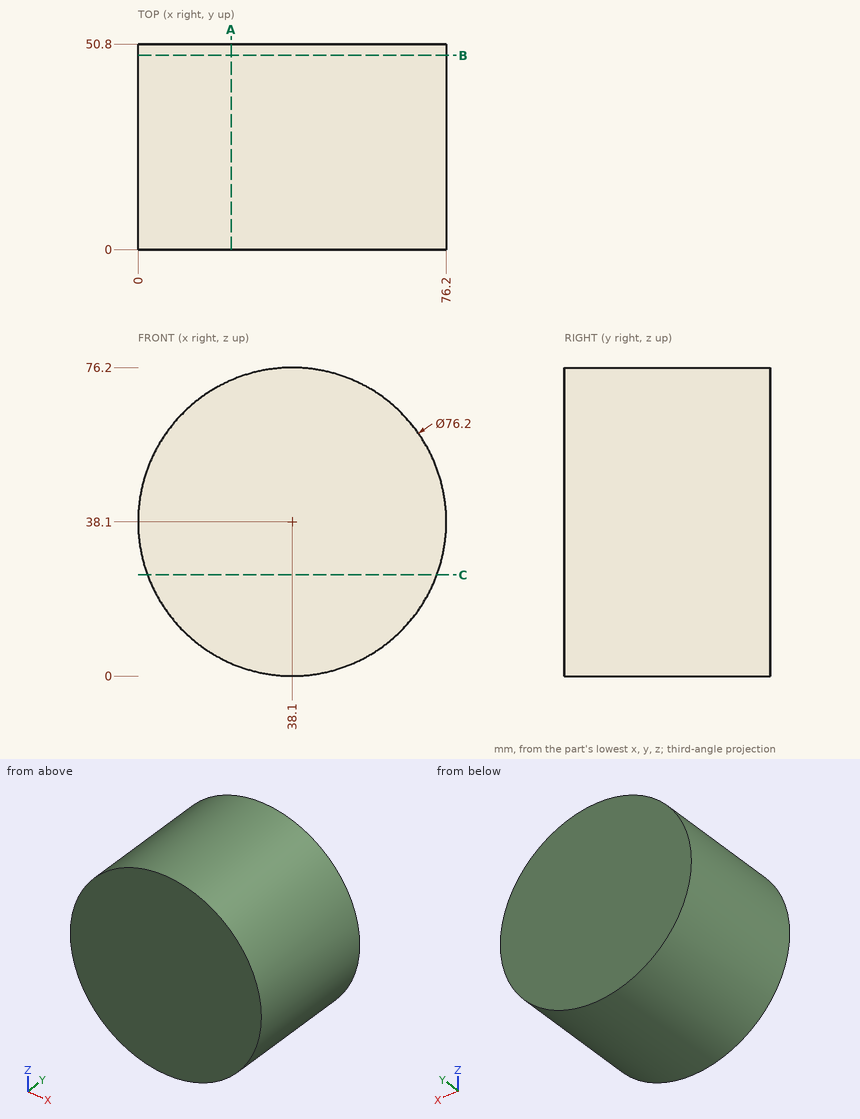
Verification items for this drawing (mm, ordinates from the low corner). Coordinates: 2 decimals unless noted, no trailing zeros. Order: outer loops, then holes, each group sorted by start corner. A loop starts at its lowest first (then second) coordinate and runs counter-clockwise, first axis right, second up. Notation, with made-up numbers: M -0.75,6.5 L 45.25,6.5 A14 ccw 45.25,26.5 Z; hole C 80.5,4.5 d10. An arc over 180 degrees is marked long. Use CSV: the item, a comma, the result in double quotes.
Item 1: Cross-section at A-A on x = 23. Record the cut outline in (y, z), then the cut area to 3 significant figures.
Returned:
outline,"M 0,3.12 L 50.8,3.12 L 50.8,73.08 L 0,73.08 Z"
area,"3,550 mm2"
Item 2: Gauge pin test, flat ends, axial feed: pin 1 Ø1.5 at (y, z) = (16, 63.5) entering from +X; pin 2 Ø2 at (y, z) = (5.5, 30.5) entering from +X; pin 3 Ø8 at (x, y) = (38, 5) entering from -Z. Record the tip position at first contact, or that the pin passes through.
Returned:
pin 1,"stops at x = 67.15"
pin 2,"stops at x = 75.62"
pin 3,"stops at z = 0"
Item 3: Cross-section at C-C on z = 25. Record the cut outline in (x, y).
Returned:
outline,"M 2.32,0 L 73.88,0 L 73.88,50.8 L 2.32,50.8 Z"
Item 4: Cross-section at B-B on y = 48. Record the cut outline in (x, z).
Returned:
outline,"C 38.1,38.1 d76.2"
Item 5: Thickness scan on line 1 along X through (y, z) = (20, 38.5); line 2 along Z through (x, y) = (42, 17); line 3 along X through (y, z) = (27, 24). Record the ranges inside material, lowest first.
Returned:
line 1,"x = 0 to 76.2"
line 2,"z = 0.2 to 76"
line 3,"x = 2.71 to 73.49"
